Job drawing, mm, ordinate dimensions from the low corner. One solid piece. A direction names the side the tool comes from. Round coordinates to 2 decimals unless told otherwise and drop trailing zeros. Order: outer loops, then holes, each group sorted by start corner. A loop starts at its lowest first (then second) coordinate and runs counter-clockwise, first axis right, second up. Notation, with made-up numbers: M 22,6 L 42,6 A9 cw 42,13 Z; hole C 23.5,-33 d3. An arc over 180 degrees is marked long. Answer as a JSON object with one key per item and string values. Group by question number.
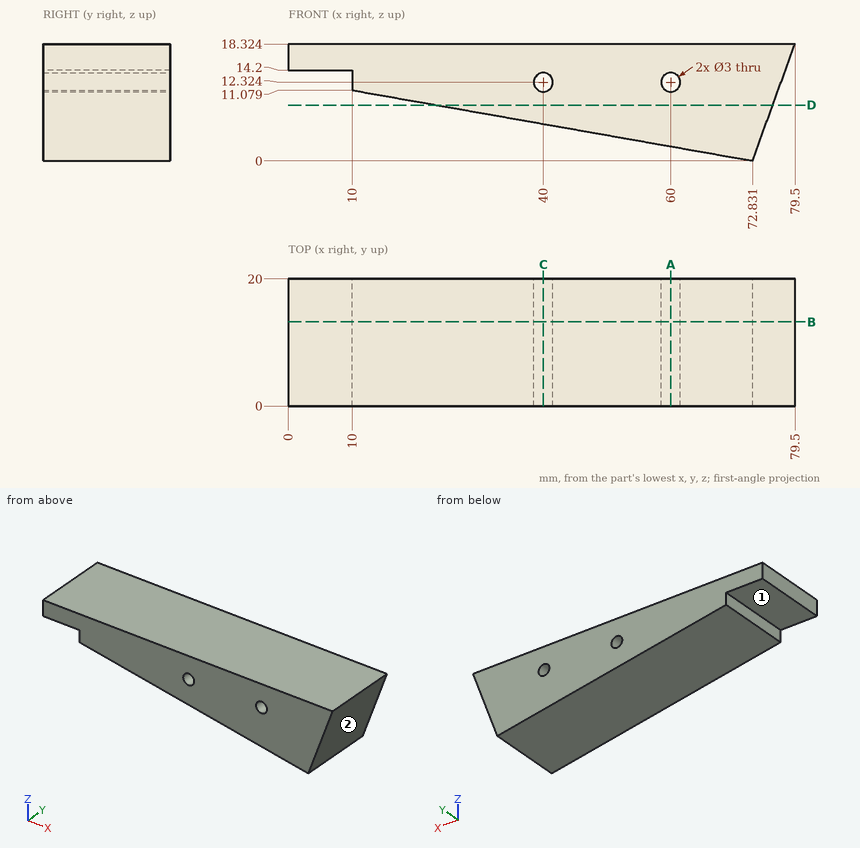
Item 1: 3-axis set-ups, long thin cutter, end or side, ignore diameter. For the marked faces 1 and 2: which of +Z, -Z, +X, -X, +Y, -Y reach the whole face in a straight line?
Item 2: Cut at D-D, the plane z = 8.75. Give the cut face in (x, y) (1 decimal).
Item 3: Flat gauge pins, fed straight in: pin 1 Ø10 at (x, z) = (48, 2.5) entering from -Y; pin 2 Ø2.5 at (x, z) = (60, 12.32) entering from -Y (3 decimals); pin 3 Ø8 at (x, y) = (5.5, 8) entering from -Z; pin 4 Ø2.5 at (y, z) = (14.5, 12.5) entering from -X. Where does each tip first touch, or does it go through?
Item 4: Cut at A-A, the plane x = 60. Give the cut face in (y, z).
Item 5: Cut at B-B, the plane y = 13.25. Give the cut face in (x, z).
Item 6: Cut at C-C, the plane x = 40. Give the cut face in (y, z).
Item 7: Drill centre lines: line 1 (X direction, y = 19, z = 13.5) (1 decimal); line 2 (X direction, y = 16.5, z = 12) (1 decimal); line 3 (Z direction, x = 7.5, y = 17.75). Where is each one in solid material? Low to high. Write a range as [from, to].
Response values:
{
 "1": {"face 1": "-Z, -X, +Y, -Y", "face 2": "-Z, +X, +Y, -Y"},
 "2": {"outline": "M 23.2,0 L 76,0 L 76,20 L 23.2,20 Z"},
 "3": {"pin 1": "y = 0", "pin 2": "through", "pin 3": "z = 14.2", "pin 4": "x = 10"},
 "4": {"outline": "M 0,2.26 L 20,2.26 L 20,10.82 L 0,10.82 Z; M 0,13.82 L 20,13.82 L 20,18.32 L 0,18.32 Z"},
 "5": {"outline": "M 0,14.2 L 10,14.2 L 10,11.08 L 72.83,0 L 79.5,18.32 L 0,18.32 Z; hole C 40,12.32 d3; hole C 60,12.32 d3"},
 "6": {"outline": "M 0,5.79 L 20,5.79 L 20,10.82 L 0,10.82 Z; M 0,13.82 L 20,13.82 L 20,18.32 L 0,18.32 Z"},
 "7": {"line 1": "[10, 39.1], [40.9, 59.1], [60.9, 77.7]", "line 2": "[10, 38.5], [41.5, 58.5], [61.5, 77.2]", "line 3": "[14.2, 18.32]"}
}
